Check sheet for the modelled part. Datum: model origin and axes. Units: mm. Face numbers are marked on the shaded views. A direction names the side the tool comes from. Round coordinates to 2 decimals unless told otherwise and drop trailing zeros. Write each loop counter-clockwise with the first axis right and the second up, starting at its lowest first coordinate (ties: lowest second). Pieces come first, ordered by that corner, then holes. Notation, with made-up numbers: (82, 29.25) -> (128, 29.25) arc R19 cw to (128, 54.25) -> close; hole circle Ø5 at (-32, 33.5). An arc over 180 degrees is marked (long way). One line per item, written item: value.
from build123d import *

# Parameters (mm, degrees)
ESTRUSIONE_ESTRUSIONE1_DEPTH = 13
ESTRUSIONE_SOTTILE5_DEPTH    = 10


# Read off the part's stored shape, not the designer's step: Estrusione-Sottile5
with BuildPart() as part:
    # Schizzo1 → Estrusione-Estrusione1 (new body)
    with BuildSketch(Plane.XY):
        with BuildLine():
            Line((32.3920487, 64.599216546), (32.3920487, 92.695802437))
            Line((32.3920487, 92.695802437), (48.470036729, 92.695802437))
            Line((48.470036729, 92.695802437), (48.470036729, 12.199228267))
            Line((48.470036729, 12.199228267), (3.151561413, 12.199228267))
            add(Edge.make_bspline(
                [(3.151561413, 12.199228267), (3.139611177, 19.224996267), (1.892686637, 31.387863298), (12.137321926, 43.966124148), (23.267751598, 47.670295467), (28.997328985, 56.366188951), (32.3920487, 61.880405589), (32.3920487, 64.599216546)],
                knots=[0, 0, 0, 0, 0.347386822, 0.514075999, 0.722780372, 0.866740614, 1, 1, 1, 1], degree=3))
        make_face()
    estrusione_estrusione1 = extrude(amount=ESTRUSIONE_ESTRUSIONE1_DEPTH)

    # Estrusione-Sottile5 outline → Estrusione-Sottile5 (add)
    with BuildSketch(Plane.XY.offset(13)):
        with BuildLine():
            Line((32.3920487, 92.695802437), (32.3920487, 64.599216546))
            add(Edge.make_bspline(
                [(32.3920487, 64.599216546), (32.3920487, 61.880405589), (28.997328985, 56.366188951), (23.267751598, 47.670295467), (12.137321926, 43.966124148), (1.892686637, 31.387863298), (3.139611177, 19.224996267), (3.151561413, 12.199228267)],
                knots=[0, 0, 0, 0, 0.133259386, 0.277219628, 0.485924001, 0.652613178, 1, 1, 1, 1], degree=3))
            Line((3.151561413, 12.199228267), (6.151557074, 12.204331005))
            add(Edge.make_bspline(
                [(6.151557074, 12.204331005), (6.149334866, 13.510808651), (6.119648943, 14.831885644), (6.06293225, 17.480029501), (6.03584378, 18.807019929), (6.037068448, 22.752005394), (6.151453161, 25.333469119), (6.757390346, 28.929919641), (7.030718923, 30.082494468), (7.57350109, 31.725152792), (7.776519692, 32.258469787), (8.231352372, 33.295835374), (8.485381605, 33.804131964), (9.889253187, 36.299307042), (11.433784909, 38.123415419), (13.69240187, 39.947060574), (14.157760625, 40.286091152), (15.150594798, 40.947311626), (15.673944983, 41.267323739), (17.308950011, 42.213099328), (18.485640453, 42.822946504), (20.909634026, 44.126845944), (22.157818902, 44.820909202), (23.995293063, 46.057426343), (24.601789725, 46.502652624), (25.48644282, 47.23845245), (25.775807333, 47.494631032), (26.331807302, 48.016372792), (26.600288227, 48.283277702), (27.899876834, 49.642128534), (28.802450288, 50.804747978), (30.05266046, 52.580806918), (30.452110657, 53.178644998), (31.036934657, 54.076643069), (31.229471218, 54.376192918), (31.61150898, 54.974569074), (31.800421327, 55.271652753), (32.379300522, 56.190094836), (32.774413439, 56.829941685), (33.536773588, 58.171274416), (33.90437134, 58.872854876), (34.558322607, 60.355334084), (34.845244987, 61.13702646), (35.262518462, 62.798404364), (35.3920487, 63.680139971), (35.3920487, 64.599216546)],
                knots=[0, 0, 0, 0, 0.0625, 0.0625, 0.125, 0.125, 0.25, 0.25, 0.3125, 0.3125, 0.34375, 0.34375, 0.375, 0.375, 0.5, 0.5, 0.53125, 0.53125, 0.5625, 0.5625, 0.625, 0.625, 0.6875, 0.6875, 0.71875, 0.71875, 0.734375, 0.734375, 0.75, 0.75, 0.8125, 0.8125, 0.84375, 0.84375, 0.859375, 0.859375, 0.875, 0.875, 0.90625, 0.90625, 0.9375, 0.9375, 0.96875, 0.96875, 1, 1, 1, 1], degree=3))
            Line((35.3920487, 64.599216546), (35.3920487, 92.695802437))
            Line((35.3920487, 92.695802437), (32.3920487, 92.695802437))
        make_face()
    estrusione_sottile5 = extrude(amount=ESTRUSIONE_SOTTILE5_DEPTH)

    # Specchia1: Estrusione-Estrusione1, Estrusione-Sottile5 across plane
    add(estrusione_estrusione1.mirror(Plane(origin=(48.470036729, 12.199228267, 13), x_dir=(0, 0, 1), z_dir=(-1, 0, 0))))
    add(estrusione_sottile5.mirror(Plane(origin=(48.470036729, 12.199228267, 13), x_dir=(0, 0, 1), z_dir=(-1, 0, 0))))


solid = part.part
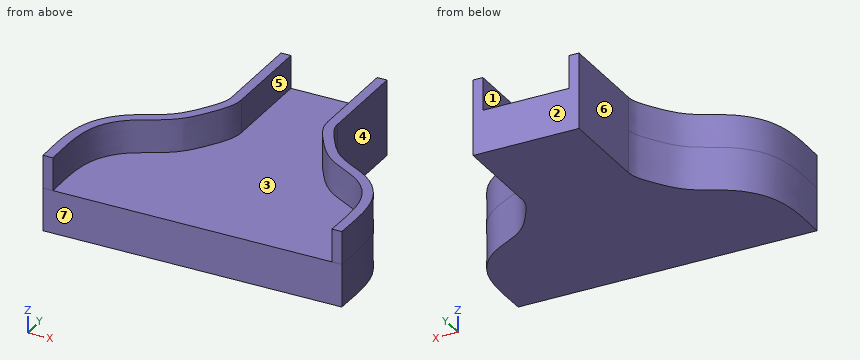
Item 1: Sectioned sample at B-B on x = 39. Enter the section's corners in (y, z), and give its area (3 significant figures).
Answer:
outline: (12.2, 0) -> (92.7, 0) -> (92.7, 13) -> (12.2, 13) -> close
area: 1,050 mm^2
Item 2: Sectioned sample at A-A on y = 78.5. Enter the section's corners in (x, z), and give its area (3 significant figures).
Answer:
outline: (32.39, 0) -> (64.55, 0) -> (64.55, 23) -> (61.55, 23) -> (61.55, 13) -> (35.39, 13) -> (35.39, 23) -> (32.39, 23) -> close
area: 478 mm^2
Item 3: Depth check by flat-ended pin: P1, Ø24, axis at x = 56.5, y = 42.5, coming from the +Z side; P2, Ø10, axis at y = 84, z = 5, coming from the +X side; P3, Ø3, axis at y = 77, z = 19, coming from the -X side. Enter the tip coordinate at first touch or a pass-through.
Answer:
P1: stops at z = 13
P2: stops at x = 64.55
P3: stops at x = 32.39
Item 4: Tool access check on the marked faces 1, 2, 3 and 4. Record the directions out of +Z, -Z, +X, -X, +Y, -Y that give a thin tool (end or side, any length) a straight path to the whole face; none if there is none.
Answer:
face 1: +Z, +Y, -Y
face 2: +Z, -Z, +X, -X, +Y
face 3: +Z, -Y
face 4: +Z, -Z, +X, +Y
Item 5: Mould release check, pull along X, two halves, no side actions. Record for the marked faces 5, 6 and 7: pulls with the +X half, pulls with the -X half, needs draft (parallel to the pull), parting line crosses it, or undercut.
Answer:
face 5: undercut
face 6: pulls with the -X half
face 7: needs draft
Item 6: Thickness scan on line 1 (X direction, y = 86.5, z = 18.75); line 2 (Z direction, x = 26.5, y = 42.5); line 3 (X direction, y = 66.5, z = 5.75). Record the ranges inside material, lowest first.
Answer:
line 1: x = 32.39 to 35.39, 61.55 to 64.55
line 2: z = 0 to 13
line 3: x = 32.39 to 64.55
